```python
from build123d import *

# Parameters (mm, degrees)
CROQUIS1_W                                           = 40
CROQUIS1_H                                           = 30
SALIENTE_EXTRUIR1_DEPTH                              = 16
CROQUIS2_R                                           = 5.1
CORTAR_EXTRUIR1_DEPTH                                = 41
REFRENTADO_PARA_TORNILLO_CON_CABEZA_HUEC_D           = 3.4
REFRENTADO_PARA_TORNILLO_CON_CABEZA_HUEC_CBORE_D     = 6.5
REFRENTADO_PARA_TORNILLO_CON_CABEZA_HUEC_CBORE_DEPTH = 3.4
DI_METRO_DE_TALADRO_4_0_4_1_D                        = 4
CROQUIS7_R                                           = 1.25
CORTAR_EXTRUIR2_DEPTH                                = 7


with BuildPart() as part:
    # Croquis1 → Saliente-Extruir1 (new body)
    with BuildSketch(Plane.XY):
        with Locations((20, 15)):
            Rectangle(CROQUIS1_W, CROQUIS1_H)
    extrude(amount=SALIENTE_EXTRUIR1_DEPTH)

    # Croquis2 → Cortar-Extruir1 (cut, through all)
    with BuildSketch(Plane(origin=(40, 0, 0), x_dir=(0, 0, -1), z_dir=(1, 0, 0))):
        with Locations((-8, 15)):
            Circle(CROQUIS2_R)
    extrude(amount=-CORTAR_EXTRUIR1_DEPTH, mode=Mode.SUBTRACT)

    # Refrentado para tornillo con cabeza hueca de M31 (through all)
    with Locations(Plane(origin=(0, 0, 0), x_dir=(-1, 0, 0), z_dir=(0, 0, -1))):
        with Locations((-5, 6), (-30, 6), (-30, 24), (-5, 24)):
            CounterBoreHole(REFRENTADO_PARA_TORNILLO_CON_CABEZA_HUEC_D / 2, REFRENTADO_PARA_TORNILLO_CON_CABEZA_HUEC_CBORE_D / 2, REFRENTADO_PARA_TORNILLO_CON_CABEZA_HUEC_CBORE_DEPTH)

    # Diámetro de taladro Ø4.0 (4)1 (through all)
    with Locations(Plane(origin=(0, 0, 0), x_dir=(-1, 0, 0), z_dir=(0, 0, -1))):
        with Locations((-16, 6), (-16, 24)):
            Hole(DI_METRO_DE_TALADRO_4_0_4_1_D / 2)

    # Croquis7 → Cortar-Extruir2 (cut)
    with BuildSketch(Plane(origin=(40, 0, 0), x_dir=(0, 0, -1), z_dir=(1, 0, 0))):
        with Locations((-8, 23)):
            Circle(CROQUIS7_R)
        with Locations((-8, 7)):
            Circle(CROQUIS7_R)
    extrude(amount=-CORTAR_EXTRUIR2_DEPTH, mode=Mode.SUBTRACT)


solid = part.part
```
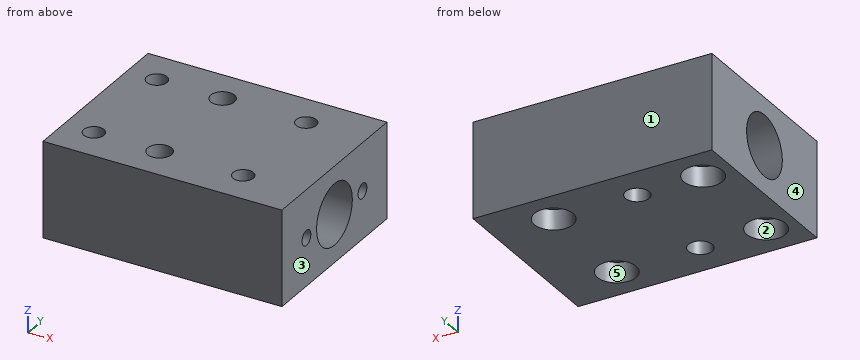
Here's how the part is built. I have some questions about the finished solid (model axes, mm). Face numbers are marked on the shaded views. A direction names the side the tool comes from. Coordinates: 2 decimals unless noted, no trailing zeros. Write each loop counter-clockwise with the first axis right and the second up, starting at its lowest first coordinate (ties: lowest second). Pieces come first, ordered by that corner, then holes. Notation, with made-up numbers: (76, -15.75) -> (135, -15.75) arc R23 ccw to (135, 11.25) -> close; hole circle Ø9 at (8, -35). An arc over 180 degrees is marked (long way). Use a Markdown table: item, result. Add a question column.
(1) If we section it at D-D, the plane x = 38: Write out the boundary of the cut face in (y, z), and give its area (3 significant figures).
(2) We'd pull the mould along X, two halves only. Please class the marked faces 1, 2 and 3: +X half, -X half, draft (parallel to the pull), parting line (faces both ways), or undercut.
(3) For the marked faces 4 and 5, which set-ups out of +Z, -Z, +X, -X, +Y, -Y let a thin tool reach every point of the face, with its end or its side?
(4) If we section it at A-A, the plane x = 16: Write out the boundary of the cut face in (y, z), and give its area (3 significant figures).
(5) If we section it at B-B, the plane z = 12.5: Write out the boundary of the cut face in (x, y).
(6) I'm going to push flat-ended pins straight in: P1, Ø2, axis at x = 5, y = 24, coming from the -Z side; P2, Ø1.5, axis at x = 34, y = 22.5, coming from the -Z side; P3, Ø2, axis at x = 29, y = 5, coming from the -Z side. Where does each tip first touch, or does it pass through?
(7) Please list where these lines run through material, in increasing order: line 1 (X direction, y = 25, z = 14); line 2 (Y direction, x = 16.5, z = 6.5); line 3 (Y direction, x = 37, z = 8).
(8) If we section it at C-C, the plane y = 15: Write out the boundary of the cut face in (x, z).
Outcome:
| question | item | result |
|---|---|---|
| 1 | outline | (0, 0) -> (30, 0) -> (30, 16) -> (0, 16) -> close; hole circle Ø2.5 at (7, 8); hole circle Ø10.2 at (15, 8); hole circle Ø2.5 at (23, 8) |
| 1 | area | 388 mm^2 |
| 2 | face 1 | draft |
| 2 | face 2 | undercut |
| 2 | face 3 | +X half |
| 3 | face 4 | +Z, -Z, -X, +Y, -Y |
| 3 | face 5 | -Z |
| 4 | outline | (0, 0) -> (4, 0) -> (4, 16) -> (0, 16) -> close; (8, 0) -> (22, 0) -> (22, 16) -> (8, 16) -> close; (26, 0) -> (30, 0) -> (30, 16) -> (26, 16) -> close; hole circle Ø10.2 at (15, 8) |
| 4 | area | 270 mm^2 |
| 5 | outline | (0, 0) -> (40, 0) -> (40, 12.6) -> (0, 12.6) -> close; (0, 17.4) -> (40, 17.4) -> (40, 30) -> (0, 30) -> close; hole circle Ø3.4 at (5, 6); hole circle Ø3.4 at (5, 24); hole circle Ø4 at (16, 6); hole circle Ø4 at (16, 24); hole circle Ø3.4 at (30, 6); hole circle Ø3.4 at (30, 24) |
| 6 | P1 | passes through |
| 6 | P2 | stops at z = 0 |
| 6 | P3 | stops at z = 3.4 |
| 7 | line 1 | x = 0 to 3.63, 6.37 to 14.27, 17.73 to 28.63, 31.37 to 40 |
| 7 | line 2 | y = 0 to 4.06, 7.94 to 10.13, 19.87 to 22.06, 25.94 to 30 |
| 7 | line 3 | y = 0 to 5.75, 8.25 to 9.9, 20.1 to 21.75, 24.25 to 30 |
| 8 | outline | (0, 0) -> (40, 0) -> (40, 2.9) -> (0, 2.9) -> close; (0, 13.1) -> (40, 13.1) -> (40, 16) -> (0, 16) -> close |
